CAD build for the part. Positions are in the model's coordinates, mm. Face numbers are marked on the shaded views. Round coordinates to 2 decimals unless told otherwise and drop trailing zeros. Order: outer loops, then holes, each group sorted by start corner. A loop starts at its lowest first (then second) coordinate and runs counter-clockwise, first axis right, second up.
```python
from build123d import *

# Parameters (mm, degrees)
SKETCH1_W           = 106
SKETCH1_H           = 121
BOSS_EXTRUDE1_DEPTH = 4
SKETCH2_W           = 100
SKETCH2_H           = 115
SKETCH2_W_2         = 97
SKETCH2_H_2         = 112
BOSS_EXTRUDE2_DEPTH = 10
SKETCH5_W           = 15
SKETCH5_H           = 15
BOSS_EXTRUDE4_DEPTH = 4
FILLET1_R           = 4
SKETCH6_R           = 2
CUT_EXTRUDE1_DEPTH  = 119
SKETCH7_R           = 2
CUT_EXTRUDE2_DEPTH  = 126
FILLET2_R           = 5


with BuildPart() as part:
    # Sketch1 → Boss-Extrude1 (new body)
    with BuildSketch(Plane(origin=(0, 0, 0), x_dir=(1, 0, 0), z_dir=(0, 1, 0))):
        Rectangle(SKETCH1_W, SKETCH1_H)
    extrude(amount=BOSS_EXTRUDE1_DEPTH)

    # Sketch2 → Boss-Extrude2 (add)
    with BuildSketch(Plane(origin=(0, 4, 0), x_dir=(1, 0, 0), z_dir=(0, 1, 0))):
        Rectangle(SKETCH2_W, SKETCH2_H)
        Rectangle(SKETCH2_W_2, SKETCH2_H_2, mode=Mode.SUBTRACT)
    extrude(amount=BOSS_EXTRUDE2_DEPTH)

    # Sketch5 → Boss-Extrude4 (add)
    with BuildSketch(Plane.XZ):
        with Locations((60.5, 1.833292933)):
            Rectangle(SKETCH5_W, SKETCH5_H)
        with Locations((-60.5, 1.833292933)):
            Rectangle(SKETCH5_W, SKETCH5_H)
    extrude(amount=-BOSS_EXTRUDE4_DEPTH)

    # Fillet1
    fillet1_edges = [part.edges().sort_by_distance(p)[0] for p in [
        (68, 2, -5.666707067),
        (68, 2, 9.333292933),
        (-68, 2, 9.333292933),
        (-68, 2, -5.666707067),
    ]]
    fillet(fillet1_edges, radius=FILLET1_R)

    # Sketch6 → Cut-Extrude1 (cut)
    with BuildSketch(Plane(origin=(53, 0, 0), x_dir=(0, 0, -1), z_dir=(1, 0, 0))):
        with Locations((40.5, 9)):
            Circle(SKETCH6_R)
        with Locations((0, 9)):
            Circle(SKETCH6_R)
        with Locations((-40.5, 9)):
            Circle(SKETCH6_R)
    extrude(amount=-CUT_EXTRUDE1_DEPTH, mode=Mode.SUBTRACT)

    # Sketch7 → Cut-Extrude2 (cut)
    with BuildSketch(Plane.XY.offset(60.5)):
        with Locations(Location((28, 9, 0), (0, 0, 180))):
            Circle(SKETCH7_R)
        with Locations(Location((-28, 9, 0), (0, 0, 180))):
            Circle(SKETCH7_R)
    extrude(amount=-CUT_EXTRUDE2_DEPTH, mode=Mode.SUBTRACT)

    # Fillet2
    fillet2_edges = [part.edges().sort_by_distance(p)[0] for p in [
        (53, 2, 60.5),
        (-53, 2, 60.5),
        (-53, 2, -60.5),
        (53, 2, -60.5),
    ]]
    fillet(fillet2_edges, radius=FILLET2_R)


solid = part.part
```
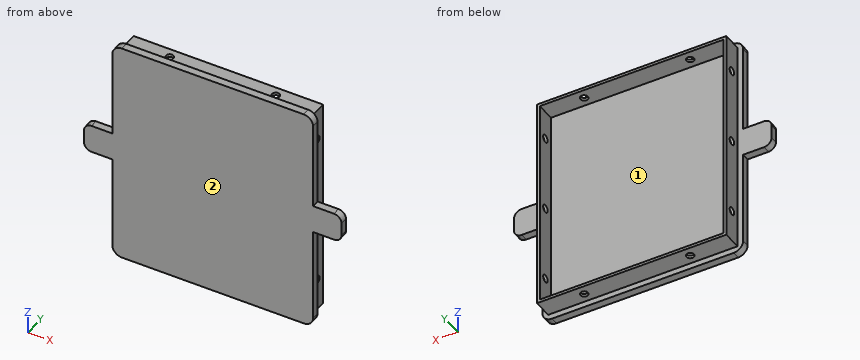
1. Cut at A-A, the plane z = -40.5. Write the cut outline in (x, y).
2. Cut at C-C, the plane y = 2.5. Write the cut outline in (x, z), and give its area (3 significant figures).
3. Drill centre lines: line 1 (X direction, y = 9, z = 57.1); line 2 (Z direction, x = 28.5, y = 6.5); line 3 (X direction, y = 8, z = -26). Where is each one in solid material? Low to high.
4. Cut at D-D, the plane y = 9. Give the number of separate pieces and of enclosed holes in the cut face, and give its area (3 significant figures).
5. Mould opens along Z. For the marked faces 1 and 2 say: released by +Z, released by -Z, zero draft, split by the parting line, or undercut.
6. Cut at B-B, the plane x = 28. Write the cut outline in (y, z).
7. Pin check, flat tips, straight feed: P1, Ø4, axis at x = -16.5, z = 27, coming from the +Y side; P2, Ø3, axis at y = 9.5, z = -25, coming from the +X side; P3, Ø4.5, axis at y = 1.5, z = -36, coming from the -X side. Stop position of each tip, or through.
Outcome:
1. outline: (-53, 0) - (53, 0) - (53, 4) - (50, 4) - (50, 7) - (48.5, 7) - (48.5, 4) - (-48.5, 4) - (-48.5, 7) - (-50, 7) - (-50, 4) - (-53, 4) - close; (-50, 11) - (-48.5, 11) - (-48.5, 14) - (-50, 14) - close; (48.5, 11) - (50, 11) - (50, 14) - (48.5, 14) - close
2. outline: (-68, -1.67) arc R4 ccw to (-64, -5.67) - (-53, -5.67) - (-53, -55.5) arc R5 ccw to (-48, -60.5) - (48, -60.5) arc R5 ccw to (53, -55.5) - (53, -5.67) - (64, -5.67) arc R4 ccw to (68, -1.67) - (68, 5.33) arc R4 ccw to (64, 9.33) - (53, 9.33) - (53, 55.5) arc R5 ccw to (48, 60.5) - (-48, 60.5) arc R5 ccw to (-53, 55.5) - (-53, 9.33) - (-64, 9.33) arc R4 ccw to (-68, 5.33) - close
2. area: 13,200 mm2
3. line 1: x = -50 to -30, -26 to 26, 30 to 50
3. line 2: z = -57.5 to -56, 56 to 57.5
3. line 3: x = -50 to -48.5, 48.5 to 50
4. separate pieces: 10
4. enclosed holes: 0
4. area: 576 mm2
5. face 1: undercut
5. face 2: zero draft
6. outline: (0, -60.5) - (4, -60.5) - (4, -57.5) - (7, -57.5) - (7, -56) - (4, -56) - (4, 56) - (7, 56) - (7, 57.5) - (4, 57.5) - (4, 60.5) - (0, 60.5) - close; (11, -57.5) - (14, -57.5) - (14, -56) - (11, -56) - close; (11, 56) - (14, 56) - (14, 57.5) - (11, 57.5) - close
7. P1: stops at y = 4
7. P2: stops at x = 50
7. P3: stops at x = -53
